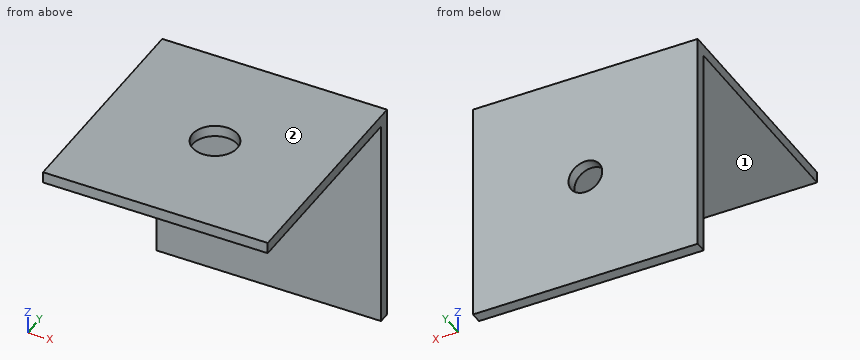
```python
from build123d import *

# Parameters (mm, degrees)
EXTRUDE_1_DEPTH     = 20
SKETCH_2_R          = 2
CUT_EXTRUDE_1_DEPTH = 35.073450075
SKETCH_3_R          = 1.5
CUT_EXTRUDE_2_DEPTH = 35.073450075


with BuildPart() as part:
    # 草图1 → 凸台-拉伸1 (new body)
    with BuildSketch(Plane(origin=(0, 0, 0), x_dir=(0, 0, -1), z_dir=(1, 0, 0))):
        Polygon((0, 0), (0, 20), (20, 20), (20, 19), (1, 19), (1, 0), align=None)
    extrude(amount=EXTRUDE_1_DEPTH)

    # 草图2 → 切除-拉伸1 (cut, through all)
    with BuildSketch(Plane(origin=(0, 0, -1), x_dir=(-1, 0, 0), z_dir=(0, 0, -1))):
        with Locations((-10, 10)):
            Circle(SKETCH_2_R)
    extrude(amount=-CUT_EXTRUDE_1_DEPTH, mode=Mode.SUBTRACT)

    # 草图3 → 切除-拉伸2 (cut, through all)
    with BuildSketch(Plane.XZ.offset(-19)):
        with Locations(Location((10, -10, 0), (0, 0, 270))):
            Circle(SKETCH_3_R)
    extrude(amount=-CUT_EXTRUDE_2_DEPTH, mode=Mode.SUBTRACT)


solid = part.part
```
Source: CAD feature listing. Evaluate the final solid. Frame: model axes, mm. Face numbers are marked on the shaded views. A direction names the side the tool comes from. Give positions to 0.01 mm unless a question says otherwise; leave off trailing zeros. Loops run counter-clockwise (first coordinate to the right, second up) from the corner with the lowest first, then second, coordinate; pieces in that order, holes last. Notation, with made-up numbers: (86, 11.5) - (104, 11.5) arc R22 cw to (104, 32.5) - close; hole circle Ø10 at (82, -30). An arc over 180 degrees is marked (long way). Use CSV: the item, a comma, the result in double quotes.
1) Cut plane A-A (x = 10). Output: boundary loops of the cut face in (y, z).
Worked out:
outline,"(0, -1) - (8, -1) - (8, 0) - (0, 0) - close; (12, -1) - (19, -1) - (19, -8.5) - (20, -8.5) - (20, 0) - (12, 0) - close; (19, -20) - (20, -20) - (20, -11.5) - (19, -11.5) - close"
2) Cut plane D-D (z = -12.25). Output: boundary loops of the cut face in (x, y), and give its area (3 significant figures).
Worked out:
outline,"(0, 19) - (20, 19) - (20, 20) - (0, 20) - close"
area,"20.0 mm^2"
3) Line query: line 1 (X direction, y = 19.2, z = -10); line 2 (Y direction, x = 10, z = -0.45); line 3 (Y direction, x = 7, z = -12.75). Output: solid intervals per line, ascending.
Worked out:
line 1,"x = 0 to 8.5, 11.5 to 20"
line 2,"y = 0 to 8, 12 to 20"
line 3,"y = 19 to 20"
4) Cut plane C-C (x = 4.75). Output: boundary loops of the cut face in (y, z), and give its area (3 significant figures).
Worked out:
outline,"(0, -1) - (19, -1) - (19, -20) - (20, -20) - (20, 0) - (0, 0) - close"
area,"39.0 mm^2"
5) Cut plane B-B (y = 10). Output: boundary loops of the cut face in (x, z), and give its area (3 significant figures).
Worked out:
outline,"(0, -1) - (8, -1) - (8, 0) - (0, 0) - close; (12, -1) - (20, -1) - (20, 0) - (12, 0) - close"
area,"16.0 mm^2"
6) Set-up query: the marked faces 1 and 2. Return all of +Z, -Z, +X, -X, +Y, -Y with unobstructed straight access to the full face (end or side cutting, diameter ignored); none if empty.
Worked out:
face 1,"-Z, +X, -X, -Y"
face 2,"+Z, +X, -X, +Y, -Y"
7) Pin query (flat end, axial travel): P1, Ø4, axis at x = 15, z = -9, coming from the -Y side; P2, Ø1.5, axis at x = 9, y = 8.5, coming from the -Z side. Return the tip coordinate at first contact, or that it passes through.
Worked out:
P1,"stops at y = 19"
P2,"stops at z = -1"
